The listing builds one solid part. Answer for the finished solid, in the listing's coordinates (mm). A direction names the side the tool comes from. Give positions to 0.01 mm unless a question says otherwise; leave off trailing zeros. Order: outer loops, then holes, each group sorted by start corner. A loop starts at its lowest first (then second) coordinate and runs counter-clockwise, first axis right, second up.
```python
from build123d import *

# Parameters (mm, degrees)
SKETCH_1_W          = 22.3
SKETCH_1_H          = 18.8
EXTRUDE_1_DEPTH     = 37.5
EXTRUDE_2_DEPTH     = 11.5
EXTRUDE_3_DEPTH     = 15
SKETCH_6_R          = 1
EXTRUDE_5_DEPTH     = 1
SKETCH_7_W          = 5
SKETCH_7_H          = 3
EXTRUDE_6_DEPTH     = 5
CUT_EXTRUDE_1_DEPTH = 12.65
SKETCH_9_R          = 1
EXTRUDE_7_DEPTH     = 8
SKETCH_10_R         = 2.5
EXTRUDE_8_DEPTH     = 8
EXTRUDE_9_DEPTH     = 23
SKETCH_12_R         = 1.5
CUT_EXTRUDE_2_DEPTH = 27.8


with BuildPart() as part:
    # 草图1 → 凸台-拉伸1 (new body)
    with BuildSketch(Plane(origin=(0, 0, 0), x_dir=(1, 0, 0), z_dir=(0, 1, 0))):
        Rectangle(SKETCH_1_W, SKETCH_1_H)
    extrude(amount=EXTRUDE_1_DEPTH)

    # 草图2 → 凸台-拉伸2 (add)
    with BuildSketch(Plane(origin=(0, 37.5, 0), x_dir=(1, 0, 0), z_dir=(0, 1, 0))):
        with BuildLine():
            Line((-5.34468737, -9.4), (5.34468737, -9.4))
            ThreePointArc((5.34468737, -9.4), (9.566941985, -5.894406054), (11.15, -0.63983183))
            ThreePointArc((11.15, -0.63983183), (9.710419772, 4.391536027), (5.827413939, 7.9))
            Line((5.827413939, 7.9), (0, 7.9))
            Line((0, 7.9), (-5.827413939, 7.9))
            ThreePointArc((-5.827413939, 7.9), (-9.536938213, 4.659739509), (-11.12855374, -0.001442574))
            ThreePointArc((-11.12855374, -0.001442574), (-11.144636924, -0.320457147), (-11.15, -0.639831856))
            ThreePointArc((-11.15, -0.639831856), (-9.566941978, -5.894406065), (-5.34468737, -9.4))
        make_face()
    extrude(amount=EXTRUDE_2_DEPTH)

    # 草图3 → 凸台-拉伸3 (add)
    with BuildSketch(Plane(origin=(0, 49, 0), x_dir=(1, 0, 0), z_dir=(0, 1, 0))):
        with BuildLine():
            Line((-5.135942831, -8.4), (5.135942831, -8.4))
            ThreePointArc((5.135942831, -8.4), (10.146278436, -0.891512764), (5.588518865, 6.9))
            Line((5.588518865, 6.9), (-5.588518865, 6.9))
            ThreePointArc((-5.588518865, 6.9), (-10.146278436, -0.891512764), (-5.135942831, -8.4))
        make_face()
    extrude(amount=EXTRUDE_3_DEPTH)

    # 草图6 → 凸台-拉伸5 (add)
    with BuildSketch(Plane(origin=(0, 64, 0), x_dir=(1, 0, 0), z_dir=(0, 1, 0))):
        with Locations((-0.226288017, -0.75)):
            Circle(SKETCH_6_R)
    extrude(amount=EXTRUDE_5_DEPTH)

    # 草图7 → 凸台-拉伸6 (add)
    with BuildSketch(Plane.XZ):
        with Locations((0, 0.75)):
            Rectangle(SKETCH_7_W, SKETCH_7_H)
    extrude(amount=EXTRUDE_6_DEPTH)

    # 草图8 → 切除-拉伸1 (cut, through all)
    with BuildSketch(Plane.XY.offset(2.25)):
        with BuildLine():
            ThreePointArc((1.5, -2.5), (0.574025149, -1.114180701), (-1.060660172, -1.439339828))
            Line((-1.060660172, -1.439339828), (1.060660172, -3.560660172))
            ThreePointArc((1.060660172, -3.560660172), (1.385819299, -3.074025149), (1.5, -2.5))
        make_face()
        with BuildLine():
            Line((1.060660172, -3.560660172), (-1.060660172, -1.439339828))
            ThreePointArc((-1.060660172, -1.439339828), (-1.060660172, -3.560660172), (1.060660172, -3.560660172))
        make_face()
    extrude(amount=-CUT_EXTRUDE_1_DEPTH, mode=Mode.SUBTRACT)

    # 草图9 → 凸台-拉伸7 (add)
    with BuildSketch(Plane(origin=(0, 0, -9.4), x_dir=(-1, 0, 0), z_dir=(0, 0, -1))):
        with BuildLine():
            Line((2.6, 11), (0, 8.4))
            ThreePointArc((0, 8.4), (-1.838477631, 9.161522369), (-2.6, 11))
            Line((-2.6, 11), (0, 13.6))
            ThreePointArc((0, 13.6), (1.838477631, 12.838477631), (2.6, 11))
        make_face()
        with Locations((0, 11)):
            Circle(SKETCH_9_R, mode=Mode.SUBTRACT)
    extrude(amount=EXTRUDE_7_DEPTH)

    # 草图10 → 凸台-拉伸8 (add)
    with BuildSketch(Plane.XY.offset(9.4)):
        with Locations((0, 11)):
            Circle(SKETCH_10_R)
    extrude(amount=EXTRUDE_8_DEPTH)

    # 草图11 → 凸台-拉伸9 (add)
    with BuildSketch(Plane(origin=(0, 64, 0), x_dir=(1, 0, 0), z_dir=(0, 1, 0))):
        with BuildLine():
            Line((-5.226288017, -6.705208095), (-5.226288017, -11.25))
            Line((-5.226288017, -11.25), (4.773711983, -11.25))
            Line((4.773711983, -11.25), (4.773711983, -6.705208095))
            ThreePointArc((4.773711983, -6.705208095), (7.549604437, -0.75), (4.773711983, 5.205208095))
            Line((4.773711983, 5.205208095), (4.773711983, 9.75))
            Line((4.773711983, 9.75), (-0.226288017, 9.75))
            Line((-0.226288017, 9.75), (-5.226288017, 9.75))
            Line((-5.226288017, 9.75), (-5.226288017, 5.205208095))
            ThreePointArc((-5.226288017, 5.205208095), (-8.002180472, -0.75), (-5.226288017, -6.705208095))
        make_face()
    extrude(amount=-EXTRUDE_9_DEPTH)

    # 草图12 → 切除-拉伸2 (cut, through all)
    with BuildSketch(Plane(origin=(0, 0, -9.4), x_dir=(-1, 0, 0), z_dir=(0, 0, -1))):
        with Locations((-8.85, 32)):
            Circle(SKETCH_12_R)
        with Locations((8.85, 32)):
            Circle(SKETCH_12_R)
    extrude(amount=-CUT_EXTRUDE_2_DEPTH, mode=Mode.SUBTRACT)


solid = part.part
```
1) Find section A-A (y = 45.5). Write down the section's boundary in (x, z).
Geometry says:
outline: (-11.15, 0.64) arc R9.51 ccw to (-11.13, 0) arc R9.51 ccw to (-5.83, -7.9) - (-5.23, -7.9) - (-5.23, -9.75) - (4.77, -9.75) - (4.77, -7.9) - (5.83, -7.9) arc R9.51 ccw to (5.34, 9.4) - (4.77, 9.4) - (4.77, 11.25) - (-5.23, 11.25) - (-5.23, 9.4) - (-5.34, 9.4) arc R9.51 ccw to start
2) Find section B-B (z = -2). Write down the section's boundary in (x, y), then the cut area to 3 significant figures.
Geometry says:
outline: (-11.15, 0) - (11.15, 0) - (11.15, 37.5) - (10.78, 37.5) - (10.78, 49) - (9.73, 49) - (9.73, 64) - (-9.73, 64) - (-9.73, 49) - (-10.78, 49) - (-10.78, 37.5) - (-11.15, 37.5) - close; hole circle Ø3 at (-8.85, 32); hole circle Ø3 at (8.85, 32)
area: 1,360 mm2
3) A tool of negligible diameter and unlimited length cuts with its end or side. For faces 4 (the cylindrical face through (-1.02, 64.49, 1.36)), 5 (the flat face through (1, -1, 2.25)), 6 (the flat face through (-10, 37.5, 7)), from which of +Z, -Z, +X, -X, +Y, -Y can it reach the whole face along a straight path? Write none if from no direction.
Geometry says:
face 4: +Y
face 5: +Z, +X, -X, -Y
face 6: +Z, -X, +Y
4) Find section D-D (y = 56.5). Write down the section's boundary in (x, z), then the cut area to 3 significant figures.
Geometry says:
outline: (-5.59, -6.9) - (-5.23, -6.9) - (-5.23, -9.75) - (4.77, -9.75) - (4.77, -6.9) - (5.59, -6.9) arc R8.51 ccw to (5.14, 8.4) - (4.77, 8.4) - (4.77, 11.25) - (-5.23, 11.25) - (-5.23, 8.36) arc R8.51 ccw to start
area: 326 mm2
5) Given P1, Ø12, axis at x = 4.5, y = 41, coming from the -Z side; P2, Ø1.5, axis at y = 56, z = 10, coming from the -X side; P3, Ø11, axis at x = -2, y = 56.5, coming from the +Z side, each flat-ended and moving along its own axis, determine where each tip first touches the part or whether it passes through.
Geometry says:
P1: stops at z = -9.75
P2: stops at x = -5.23
P3: stops at z = 11.25
6) For a pull along Y with two mould halves and no side action, classify faces 1 (the cylindrical face through (1.818, 9.141, -13.344)), 2 (the cylindrical face through (-9.54, 30.67, -0.13)), 3 (the cylindrical face through (10.14, 56.4, 1.02)) as +Y half, -Y half, draft (parallel to the pull), parting line (faces both ways), or undercut.
Geometry says:
face 1: -Y half
face 2: undercut
face 3: draft
7) Straight lines are drawn through the part: probe 1 along Y at (x, z) = (-8.85, 1); probe 2 along Z at (x, y) = (1.5, -1.5); probe 3 along Z at (x, y) = (-1, 38). For each, find the intervals that lie inside material, in ascending order.
Geometry says:
probe 1: y = 0 to 30.5, 33.5 to 64
probe 2: z = -0.75 to 2.25
probe 3: z = -7.9 to 9.4
8) Find section C-C (x = 8.85). Write down the section's boundary in (y, z), then the cut area to 3 significant figures.
Geometry says:
outline: (0, -9.4) - (30.5, -9.4) - (30.5, 9.4) - (0, 9.4) - close; (33.5, -9.4) - (37.5, -9.4) - (37.5, -5.56) - (49, -5.56) - (49, -3.88) - (64, -3.88) - (64, 5.16) - (49, 5.16) - (49, 6.84) - (37.5, 6.84) - (37.5, 9.4) - (33.5, 9.4) - close
area: 927 mm2
